Geometry: see drawing. Coordinates: mm, zero at the bounding-box minimum. Give positions to 0.01 mm unless a question says otherwise; leave off trailing zeros. Order: outer loops, then holes, each group sorted by start corner. A loop starts at its lowest first (then second) coordinate and runs counter-clockwise, first axis right, second up. Notation, with made-up numbers: M 73,48.25 L 91,48.25 A22 ccw 91,57.25 Z; hole C 78.25,-15 d6. An arc over 180 degrees is marked long. Use a Markdown table: item, result.
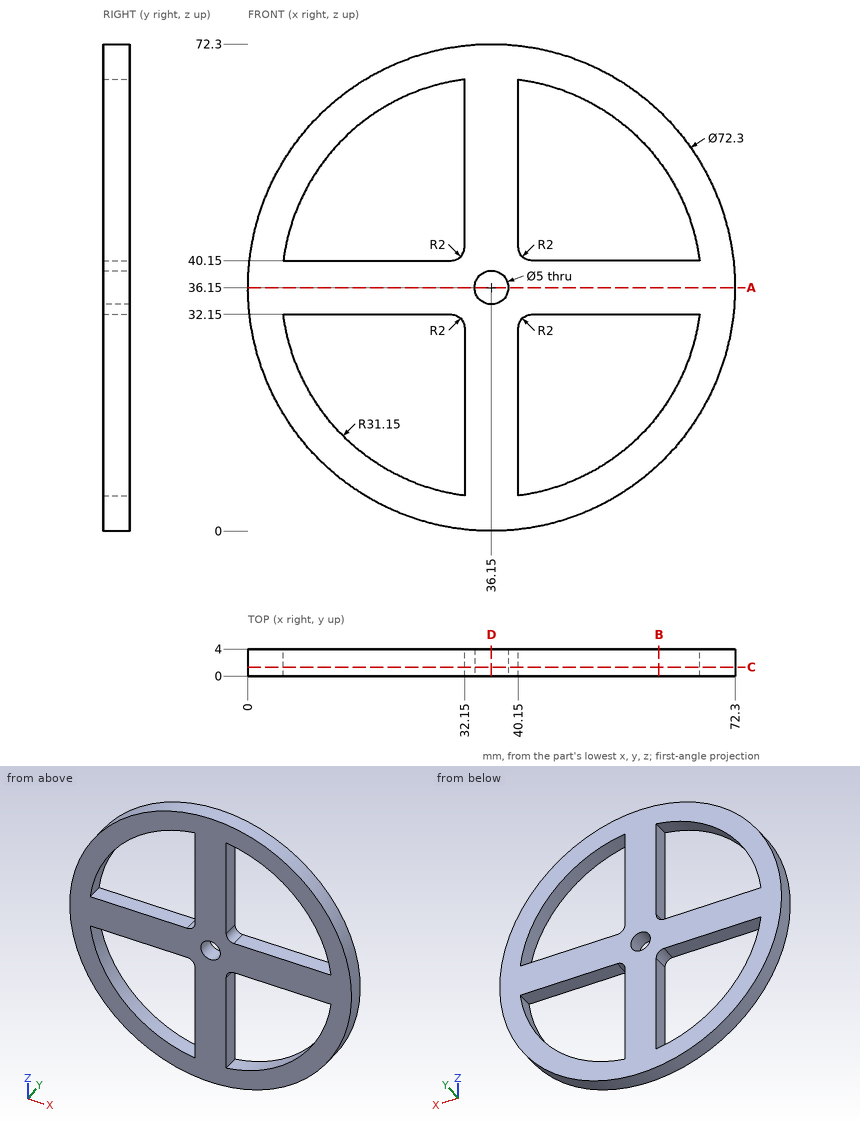
1) Cut plane B-B on x = 61. Return loops of the section in (y, z), and give its area (3 significant figures).
Response values:
| item | result |
|---|---|
| outline | M 0,9.9 L 4,9.9 L 4,17.37 L 0,17.37 Z; M 0,32.15 L 4,32.15 L 4,40.15 L 0,40.15 Z; M 0,54.93 L 4,54.93 L 4,62.4 L 0,62.4 Z |
| area | 91.8 mm² |
2) Cut plane C-C on y = 1.3. Return loops of the section in (x, z), and give its area (3 significant figures).
Response values:
| item | result |
|---|---|
| outline | C 36.15,36.15 d72.3; hole M 5.26,32.15 A31.15 ccw 32.15,5.26 L 32.15,30.15 A2 ccw 30.15,32.15 Z; hole M 5.26,40.15 L 30.15,40.15 A2 ccw 32.15,42.15 L 32.15,67.04 A31.15 ccw Z; hole C 36.15,36.15 d5; hole M 40.15,5.26 A31.15 ccw 67.04,32.15 L 42.15,32.15 A2 ccw 40.15,30.15 Z; hole M 40.15,42.15 A2 ccw 42.15,40.15 L 67.04,40.15 A31.15 ccw 40.15,67.04 Z |
| area | 1,970 mm² |
3) Cut plane D-D on x = 36.15. Return loops of the section in (y, z).
Response values:
| item | result |
|---|---|
| outline | M 0,0 L 4,0 L 4,33.65 L 0,33.65 Z; M 0,38.65 L 4,38.65 L 4,72.3 L 0,72.3 Z |
4) First-contact query: pin 1 Ø4 at (x, z) = (8.5, 29.5) entering from +Y; pin 2 Ø1.2 at (y, z) = (3, 49) entering from +X; pin 3 Ø2 at (x, y) = (15, 1) entering from +Z; pin 4 Ø1.5 at (x, y) = (10.5, 1) entering from -Z. Flat tips, straight axial feed; report the tip coordinate or a pass-through.
Response values:
| item | result |
|---|---|
| pin 1 | passes through |
| pin 2 | stops at x = 70.16 |
| pin 3 | stops at z = 66.16 |
| pin 4 | stops at z = 9.94 |
5) Cut plane A-A on z = 36.15. Return loops of the section in (x, y), and give its area (3 significant figures).
Response values:
| item | result |
|---|---|
| outline | M 0,0 L 33.65,0 L 33.65,4 L 0,4 Z; M 38.65,0 L 72.3,0 L 72.3,4 L 38.65,4 Z |
| area | 269 mm² |
6) Material intervals for line 1 (X direction, y = 1.6, z = 36.15); line 2 (Z direction, x = 27.5, y = 2.5); line 3 (Z direction, x = 54, y = 3.85), sorted ascending. Write a range as from..to.
Response values:
| item | result |
|---|---|
| line 1 | x = 0..33.65, 38.65..72.3 |
| line 2 | z = 1.05..6.23, 32.15..40.15, 66.07..71.25 |
| line 3 | z = 4.71..10.62, 32.15..40.15, 61.68..67.59 |
